from build123d import *

# Parameters (mm, degrees)
SKETCH2_R                      = 78.359
SKETCH2_R_2                    = 76.3651
BOSS_EXTRUDE1_DEPTH            = 635
SKETCH4_R                      = 3.2639
CUT_EXTRUDE2_DEPTH             = 79.359
CIRPATTERN2_COUNT              = 4
CUT_EXTRUDE3_REACH             = 191.175
SKETCH5_R                      = 2.57937
CUT_EXTRUDE3_DIRECTION_2_DEPTH = 33.457360675
VENT_HOLE_REACH                = 191.175
SKETCH6_R                      = 3.175
F_4_CLEARANCE_HOLE1_D          = 3.2639
CIRPATTERN3_COUNT              = 2
CIRPATTERN3_ANGLE              = 90


with BuildPart() as part:
    # Sketch2 → Boss-Extrude1 (new body)
    with BuildSketch(Plane(origin=(0, 0, 0), x_dir=(1, 0, 0), z_dir=(0, 1, 0))):
        Circle(SKETCH2_R)
        Circle(SKETCH2_R_2, mode=Mode.SUBTRACT)
    extrude(amount=BOSS_EXTRUDE1_DEPTH)

    # Sketch4 → Cut-Extrude2 (cut, symmetric)
    with BuildSketch(Plane.XY):
        with Locations((0, 449.5038)):
            Circle(SKETCH4_R)
    cut_extrude2 = extrude(amount=CUT_EXTRUDE2_DEPTH, both=True, mode=Mode.SUBTRACT)

    # CirPattern2: Cut-Extrude2 ×4 about axis
    cirpattern2_axis = Axis((0, 635, 0), (0, 1, 0))
    for i in range(1, CIRPATTERN2_COUNT):
        add(cut_extrude2.rotate(cirpattern2_axis, i * 360 / CIRPATTERN2_COUNT), mode=Mode.SUBTRACT)

    # Sketch5 → Cut-Extrude3 (cut, up to next)
    with BuildSketch(Plane(origin=(55.408180267, 0, 55.408180267), x_dir=(0, -1, 0), z_dir=(0.707106781, 0, 0.707106781)), mode=Mode.PRIVATE) as cut_extrude3_sk1:
        with Locations((-449.5038, 0)):
            Circle(SKETCH5_R)
    cut_extrude3_tool1 = extrude(cut_extrude3_sk1.sketch, amount=-CUT_EXTRUDE3_REACH, mode=Mode.PRIVATE) & part.part
    add(cut_extrude3_tool1.solids().sort_by_distance((55.40818, 449.5038, 55.40818))[0], mode=Mode.SUBTRACT)

    # Sketch5 → Cut-Extrude3 direction 2 (cut)
    with BuildSketch(Plane(origin=(55.408180267, 0, 55.408180267), x_dir=(0, -1, 0), z_dir=(0.707106781, 0, 0.707106781))):
        with Locations((-449.5038, 0)):
            Circle(SKETCH5_R)
    extrude(amount=CUT_EXTRUDE3_DIRECTION_2_DEPTH, mode=Mode.SUBTRACT)

    # Sketch6 → Vent Hole (cut, up to next)
    with BuildSketch(Plane(origin=(189.175360534, 0, -78.359), x_dir=(-0.707106781, 0, 0.707106781), z_dir=(-0.707106781, 0, -0.707106781)), mode=Mode.PRIVATE) as vent_hole_sk1:
        with Locations((189.175360534, 304.8)):
            Circle(SKETCH6_R)
    vent_hole_tool1 = extrude(vent_hole_sk1.sketch, amount=VENT_HOLE_REACH, mode=Mode.PRIVATE) & part.part
    add(vent_hole_tool1.solids().sort_by_distance((55.40818, 304.8, 55.40818))[0], mode=Mode.SUBTRACT)

    # #4 Clearance Hole1 (through all)
    with Locations(Plane.XY.offset(78.359)):
        with Locations((0, 76.2)):
            f_4_clearance_hole1 = Hole(F_4_CLEARANCE_HOLE1_D / 2)

    # CirPattern3: #4 Clearance Hole1 ×2 about axis
    cirpattern3_axis = Axis((0, 0, 0), (0, 1, 0))
    for i in range(1, CIRPATTERN3_COUNT):
        add(f_4_clearance_hole1.rotate(cirpattern3_axis, i * CIRPATTERN3_ANGLE / (CIRPATTERN3_COUNT - 1)), mode=Mode.SUBTRACT)


solid = part.part
Verification items for the finished model (mm, model axes). Coordinates: 2 decimals unless noted, no trailing zeros. Order: outer loops, then holes, each group sorted by start corner. A loop starts at its lowest first (then second) coordinate and runs counter-clockwise, first axis right, second up.
1. Release check for a two-part mould opening along X. For faces 1 (the face through (17, 635, 75)), 2 (the face through (74.74, 313.06, -23.54)), 3 (the face through (41.053, 313.055, -64.391)) record: +X half, -X half, draft (parallel to the pull), parting line (faces both ways), or undercut.
Results found:
face 1: draft
face 2: parting line
face 3: undercut
2. Go/stop test with flat-tipped pins: pin 1 Ø12 at (y, z) = (94.5, 38.5) entering from -X; pin 2 Ø2 at (y, z) = (186.5, 53.5) entering from -X; pin 3 Ø10 at (x, y) = (-23, 335.5) entering from +Z. Record where each tip stops, or that it passes through.
Results found:
pin 1: stops at x = -71.3
pin 2: stops at x = -58.17
pin 3: stops at z = 76.26
3. Sectioned sample at A-A, the plane x = -23. Record the cut outline in (y, z).
Results found:
outline: (0, -74.91) - (635, -74.91) - (635, -72.82) - (0, -72.82) - close; (0, 72.82) - (635, 72.82) - (635, 74.91) - (0, 74.91) - close
4. Sectioned sample at B-B, the plane z = 42. Record the cut outline in (x, y).
Results found:
outline: (-66.15, 0) - (-63.78, 0) - (-63.78, 635) - (-66.15, 635) - close; (63.78, 0) - (66.15, 0) - (66.15, 635) - (63.78, 635) - close
5. Sectioned sample at C-C, the plane y = 532. Record the cut outline in (x, z), and give its area (3 significant figures).
Results found:
outline: circle Ø156.72 at (0, 0); hole circle Ø152.73 at (0, 0)
area: 969 mm2
6. Scan lines: line 1 (Y direction, x = 77.35, z = 0); line 2 (X direction, y = 367.5, z = 3); line 3 (Z direction, x = 0, y = 204). Record each from-to range of solid material in increasing order.
Results found:
line 1: y = 0 to 74.57, 77.83 to 446.24, 452.77 to 635
line 2: x = -78.3 to -76.31, 76.31 to 78.3
line 3: z = -78.36 to -76.37, 76.37 to 78.36
